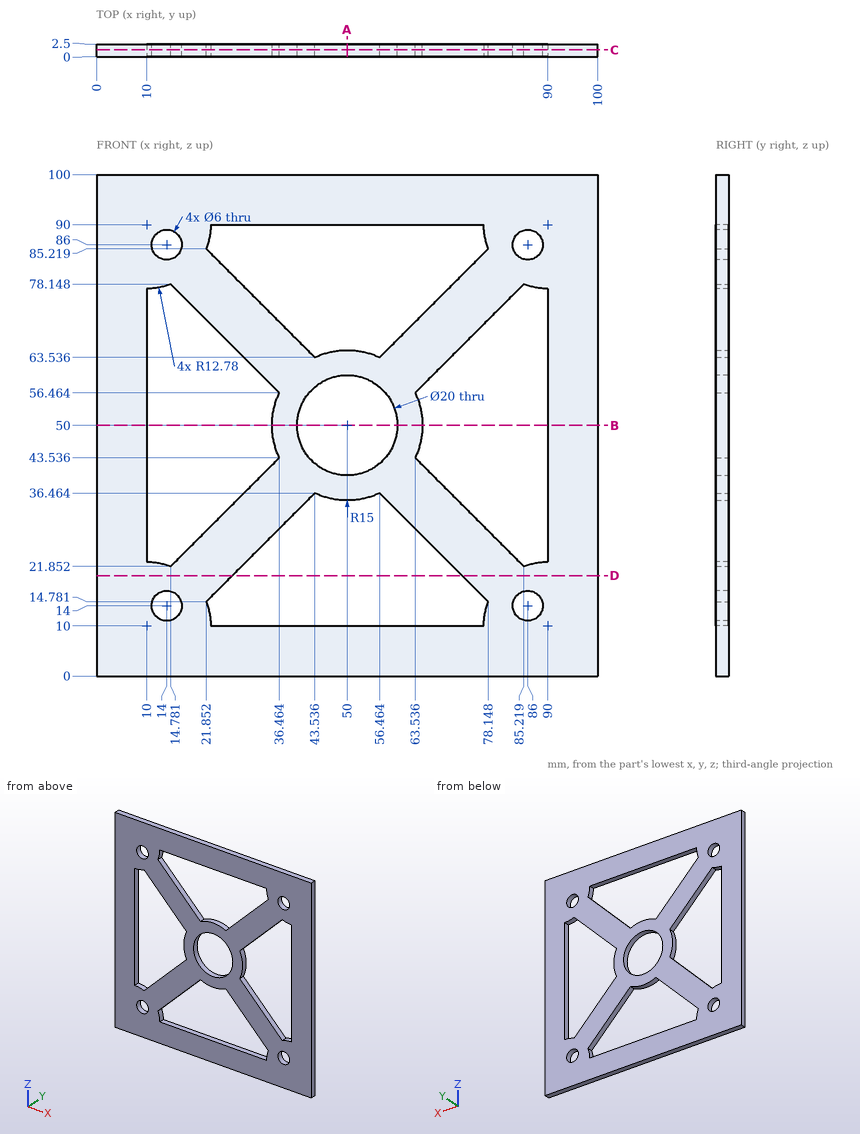
Answer from the drawing. Dimensions are ordinates in mm from the lowest x, y and z of the part. Give positions to 0.01 mm unless a question says otherwise; leave off trailing zeros. Order: outer loops, then holes, each group sorted by start corner. A loop starts at its lowest first (then second) coordinate and runs counter-clockwise, first axis right, second up. Notation, with made-up numbers: (59, -4.75) -> (84, -4.75) arc R15 ccw to (84, 19.25) -> close; hole circle Ø10 at (14, -1.75). An arc over 180 degrees is marked (long way). Answer as a JSON object with one key per item and string values. Group by question number.
1. Section C-C on y = 1.35 is taken. Count the separate pieces of the cut face and the enclosed holes in it, plus the area to 3 significant figures.
2. Section A-A on x = 50 is taken. Determine the outline of the cut face in (y, z).
3. Consider line 1 along X through (y, z) = (0.5, 53); line 2 along Z through (x, y) = (46.5, 1.2) (1 decimal); line 3 along Z through (x, y) = (66.5, 1.7). Determine where each line is inside the solid, lowest interval first. Write a range as [from, to].
4. Section B-B on z = 50 is taken. Determine the outline of the cut face in (x, y).
5. Section D-D on z = 20 is taken. Determine the outline of the cut face in (x, y).
6. A flat-ended cylindrical pin translates along its axis: pin 1 Ø5 at (x, z) = (14, 86) entering from +Y. Find the tip coordinate at first contact, or state that the pin passes through.
Result sheet:
{
 "1": {"separate pieces": "1", "enclosed holes": "9", "area": "5,570 mm^2"},
 "2": {"outline": "(0, 0) -> (2.5, 0) -> (2.5, 10) -> (0, 10) -> close; (0, 35) -> (2.5, 35) -> (2.5, 40) -> (0, 40) -> close; (0, 60) -> (2.5, 60) -> (2.5, 65) -> (0, 65) -> close; (0, 90) -> (2.5, 90) -> (2.5, 100) -> (0, 100) -> close"},
 "3": {"line 1": "x = [0, 10], [35.3, 40.46], [59.54, 64.7], [90, 100]", "line 2": "z = [0, 10], [35.4, 40.6], [59.4, 64.6], [90, 100]", "line 3": "z = [0, 10], [26.43, 40.57], [59.43, 73.57], [90, 100]"},
 "4": {"outline": "(0, 0) -> (10, 0) -> (10, 2.5) -> (0, 2.5) -> close; (35, 0) -> (40, 0) -> (40, 2.5) -> (35, 2.5) -> close; (60, 0) -> (65, 0) -> (65, 2.5) -> (60, 2.5) -> close; (90, 0) -> (100, 0) -> (100, 2.5) -> (90, 2.5) -> close"},
 "5": {"outline": "(0, 0) -> (27.07, 0) -> (27.07, 2.5) -> (0, 2.5) -> close; (72.93, 0) -> (100, 0) -> (100, 2.5) -> (72.93, 2.5) -> close"},
 "6": {"pin 1": "passes through"}
}
